Source: CAD feature listing. Evaluate the final solid. Frame: model axes, mm. A direction names the side the tool comes from. Round coordinates to 2 decimals unless told otherwise and drop trailing zeros. Order: outer loops, then holes, each group sorted by start corner. A loop starts at its lowest first (then second) coordinate and runs counter-clockwise, first axis right, second up. Notation, with made-up numbers: (44.5, 75) - (68.5, 75) arc R21 cw to (68.5, 97) - close; hole circle Ø4 at (-8, 16.25). An arc over 180 degrees is marked (long way). Put each result on its own line as item: value. Start each with the question number.
1) Contact query for flat-ended pins moving along their axis: P1, Ø12, axis at x = 148, z = 83.5, coming from the -Y side; P2, Ø8, axis at y = -75, z = 56, coming from the -X side; P3, Ø8, axis at x = 141, z = 86, coming from the +Y side. Output: stop coordinate, or through.
2) Line query: probe 1 along X at (y, z) = (201, 38); probe 2 along Y at (x, z) = (76.5, 76.5); probe 3 along Y at (x, z) = (127, 41.5). Output: solid intervals per line, ascending. Write a range as [from, to].
3) Section A-A on z = 92.5. Output: boundary loops of the cut face in (x, y), then the cut area to 3 significant figures.
4) Section C-C on x = 167. Output: boundary loops of the cut face in (y, z).
5) Access query for faces 1 (the face through (136, 24, 0)), 2 (the face through (176.53, -197, 50)), 3 (the face through (67.31, 253, 50)). Directions: +Z, -Z, +X, -X, +Y, -Y. A direction counts if a zero-diameter tool reaches every point of the face in a straight line with its end or side. Return the directions, or none.
6) Section B-B on y = -142. Output: boundary loops of the cut face in (x, z), then the cut area to 3 significant figures.
```python
from build123d import *

# Parameters (mm, degrees)
BOSS_EXTRUDE1_DEPTH = 101.6


with BuildPart() as part:
    # Sketch1 → Boss-Extrude1 (new body)
    with BuildSketch(Plane.XY):
        with BuildLine():
            Line((60.96, 197.131308881), (60.96, 307.367308881))
            Line((60.96, 307.367308881), (67.31, 307.367308881))
            Line((67.31, 307.367308881), (67.31, 197.400739769))
            ThreePointArc((67.31, 197.400739769), (68.305399944, 187.9124022), (71.248256772, 178.837218205))
            Line((71.248256772, 178.837218205), (178.504159142, -62.568409333))
            ThreePointArc((178.504159142, -62.568409333), (181.774000062, -72.651947106), (182.88, -83.194544404))
            Line((182.88, -83.194544404), (182.88, -307.367308881))
            Line((182.88, -307.367308881), (176.53, -307.367308881))
            Line((176.53, -307.367308881), (176.53, -83.463975292))
            ThreePointArc((176.53, -83.463975292), (175.534600056, -73.975637723), (172.591743228, -64.900453728))
            Line((172.591743228, -64.900453728), (65.335840858, 176.50517381))
            ThreePointArc((65.335840858, 176.50517381), (62.065999938, 186.588711582), (60.96, 197.131308881))
        make_face()
    extrude(amount=BOSS_EXTRUDE1_DEPTH)


solid = part.part
```
Answer sheet:
1. P1: y = -23.06
1. P2: x = 174.8
1. P3: y = 30.85
2. probe 1: [60.96, 67.31]
2. probe 2: [151.38, 167.02]
2. probe 3: [37.71, 53.35]
3. outline: (60.96, 197.13) arc R50.8 ccw to (65.34, 176.51) - (172.59, -64.9) arc R45.72 cw to (176.53, -83.46) - (176.53, -307.37) - (182.88, -307.37) - (182.88, -83.19) arc R50.8 ccw to (178.5, -62.57) - (71.25, 178.84) arc R45.72 cw to (67.31, 197.4) - (67.31, 307.37) - (60.96, 307.37) - close
3. area: 4,060 mm^2
4. outline: (-52.31, 0) - (-36.68, 0) - (-36.68, 101.6) - (-52.31, 101.6) - close
5. face 1: -Z, +X, -X, +Y, -Y
5. face 2: +Z, -Z, -X, -Y
5. face 3: +Z, -Z, +X, +Y
6. outline: (176.53, 0) - (182.88, 0) - (182.88, 101.6) - (176.53, 101.6) - close
6. area: 645 mm^2
